Could you check a few things on this drawing? It's one solid part, dimensions in mm from its lowest x, y, z. A direction names the side the tool comes from. Coordinates: 2 decimals unless noted, no trailing zeros. Write each loop counter-clockwise with the first axis right and the second up, starting at its lowest first coordinate (ties: lowest second). Pieces come first, ordered by that corner, then holes. Notation, with made-up numbers: (35, 23) - (80, 23) arc R27 cw to (80, 39) - close; hole circle Ø11 at (-24, -7). An arc over 180 degrees is marked (long way). Write each question's results on one line, items separated by ' | '. Start each with the question number.
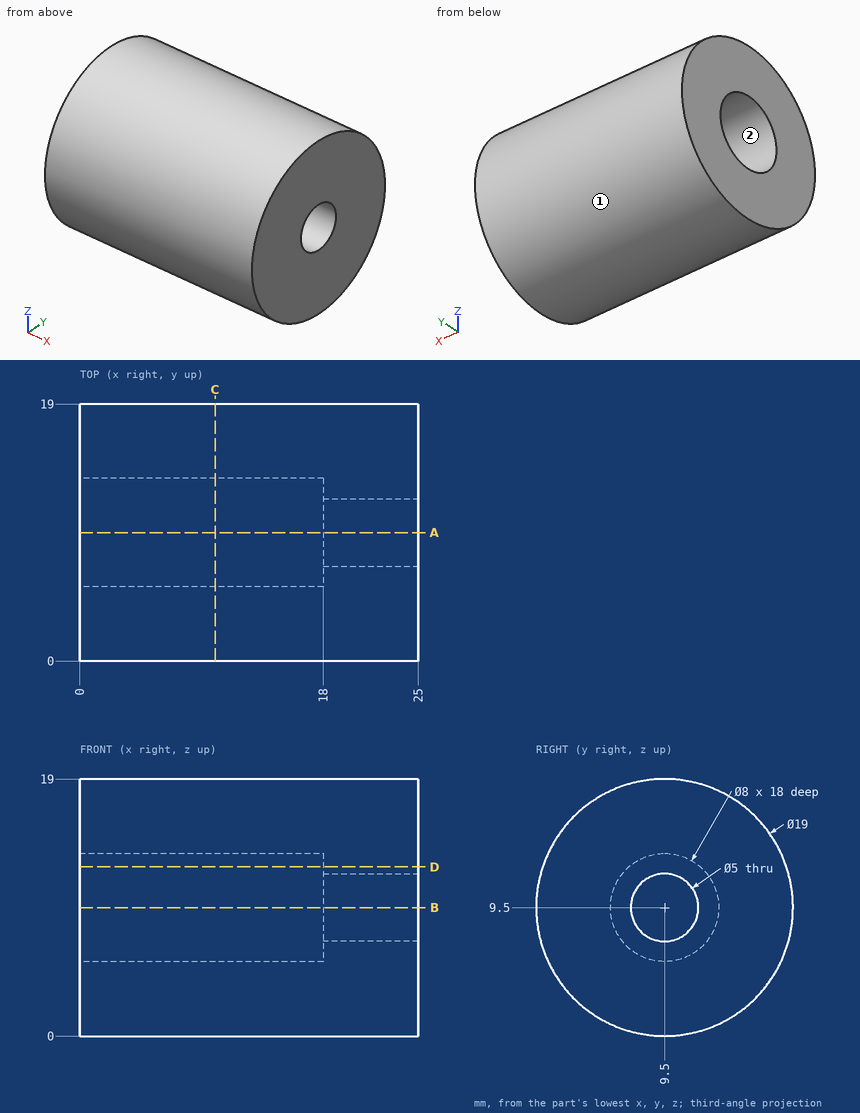
Q1. If we section it at C-C (x = 10): Please give me the cut outline in (y, z).
Q2. If we section it at A-A (y = 9.5): Please give me the cut outline in (x, z), then the cut area to 3 significant figures.
Q3. I'm going to push flat-ended pins straight in: pin 1 Ø10 at (x, z) = (4, 13.5) entering from -Y; pin 2 Ø3 at (x, z) = (11.5, 4) entering from -Y; pin 3 Ø5 at (x, y) = (10, 13) entering from -Z; pin 4 Ø5 at (x, y) = (13.5, 12.5) entering from +Z. Where does each tip first touch, or does it pass through?
Q4. I need wall thicknesses on line 1 along Y through (x, z) = (9.5, 9.5); line 2 along Y through (x, z) = (14, 12); line 3 along Z through (x, y) = (12.25, 9.25). Which ranges of each line are inside material? Lowest first, please. Write a range as from..to.
Q5. If we section it at D-D (z = 12.5): Please give me the cut outline in (x, y), then the cut area to 3 significant figures.
Q6. For the marked faces 1 and 2, which set-ups out of +Z, -Z, +X, -X, +Y, -Y let a thin tool reach every point of the face, with its end or its side?
Answer list:
1) outline: circle Ø19 at (9.5, 9.5); hole circle Ø8 at (9.5, 9.5)
2) outline: (0, 0) - (25, 0) - (25, 7) - (18, 7) - (18, 5.5) - (0, 5.5) - close; (0, 13.5) - (18, 13.5) - (18, 12) - (25, 12) - (25, 19) - (0, 19) - close | area: 296 mm2
3) pin 1: stops at y = 0 | pin 2: stops at y = 0.88 | pin 3: stops at z = 0.05 | pin 4: stops at z = 18.99
4) line 1: y = 0..5.5, 13.5..19 | line 2: y = 0.33..6.38, 12.62..18.67 | line 3: z = 0..5.51, 13.49..19
5) outline: (0, 0.49) - (25, 0.49) - (25, 18.51) - (0, 18.51) - (0, 12.15) - (18, 12.15) - (18, 6.85) - (0, 6.85) - close | area: 355 mm2
6) face 1: +X, -X | face 2: -X
